from build123d import *

# Parameters (mm, degrees)
SKETCH2_R             = 19
BOSS_EXTRUDE1_DEPTH   = 5
SKETCH3_R             = 5
CUT_EXTRUDE1_DEPTH    = 43.679034666
SKETCH4_R             = 4
CUT_EXTRUDE2_DEPTH    = 43.679034666
M4X0_7_TAPPED_HOLE1_D = 3.3
CUT_EXTRUDE3_DEPTH    = 6.43
CIRPATTERN1_COUNT     = 4


with BuildPart() as part:
    # Sketch1 → Revolve1 (revolve)
    with BuildSketch(Plane(origin=(0, 0, 0), x_dir=(0, 0, -1), z_dir=(1, 0, 0)), mode=Mode.PRIVATE) as revolve1_sk:
        Polygon((0, 9), (0, 6.15), (26.545687362, 6.15), (28.453012328, 0), (29.5, 0), (27.011788484, 8.023017104), (25.5, 9), align=None)
    revolve(revolve1_sk.sketch.rotate(Axis((0, 9, 0), (0, -1, 0)), 180), axis=Axis((0, 9, 0), (0, -1, 0)))

    # Sketch2 → Boss-Extrude1 (add)
    with BuildSketch(Plane.XZ.offset(-6.15)):
        with Locations(Location((0, 0, 0), (0, 0, 90))):
            Circle(SKETCH2_R)
    extrude(amount=BOSS_EXTRUDE1_DEPTH)

    # Sketch3 → Cut-Extrude1 (cut, through all)
    with BuildSketch(Plane(origin=(0, 9, 0), x_dir=(1, 0, 0), z_dir=(0, 1, 0))):
        with Locations(Location((0, 19, 0), (0, 0, 270))):
            Circle(SKETCH3_R)
        with Locations(Location((19, 0, 0), (0, 0, 270))):
            Circle(SKETCH3_R)
        with Locations(Location((0, -19, 0), (0, 0, 270))):
            Circle(SKETCH3_R)
        with Locations(Location((-19, 0, 0), (0, 0, 270))):
            Circle(SKETCH3_R)
    extrude(amount=-CUT_EXTRUDE1_DEPTH, mode=Mode.SUBTRACT)

    # Sketch4 → Cut-Extrude2 (cut, through all)
    with BuildSketch(Plane(origin=(0, 9, 0), x_dir=(1, 0, 0), z_dir=(0, 1, 0))):
        with Locations(Location((0, 0, 0), (0, 0, 270))):
            Circle(SKETCH4_R)
    extrude(amount=-CUT_EXTRUDE2_DEPTH, mode=Mode.SUBTRACT)

    # M4x0.7 Tapped Hole1 (through all)
    with Locations(Plane(origin=(0, 9, 0), x_dir=(1, 0, 0), z_dir=(0, 1, 0))):
        with Locations((-15.556349186, 15.556349186), (15.556349186, 15.556349186), (15.556349186, -15.556349186), (-15.556349186, -15.556349186)):
            Hole(M4X0_7_TAPPED_HOLE1_D / 2)

    # Sketch9 → Cut-Extrude3 (cut)
    with BuildSketch(Plane.XY.offset(-29.5)):
        with BuildLine():
            Line((-9.875, 6.636508552), (9.875, 6.636508552))
            ThreePointArc((9.875, 6.636508552), (12.5, 4.011508552), (9.875, 1.386508552))
            Line((9.875, 1.386508552), (-9.875, 1.386508552))
            ThreePointArc((-9.875, 1.386508552), (-12.5, 4.011508552), (-9.875, 6.636508552))
        make_face()
    cut_extrude3 = extrude(amount=CUT_EXTRUDE3_DEPTH, mode=Mode.SUBTRACT)

    # CirPattern1: Cut-Extrude3 ×4 about axis
    cirpattern1_axis = Axis((0, 0, 0), (0, 1, 0))
    for i in range(1, CIRPATTERN1_COUNT):
        add(cut_extrude3.rotate(cirpattern1_axis, i * 360 / CIRPATTERN1_COUNT), mode=Mode.SUBTRACT)


solid = part.part
Build history of the part. All positions in model axes, mm. A direction names the side the tool comes from. Give positions to 0.01 mm unless a question says otherwise; leave off trailing zeros. Order: outer loops, then holes, each group sorted by start corner. A loop starts at its lowest first (then second) coordinate and runs counter-clockwise, first axis right, second up. Notation, with made-up numbers: M 10,2.5 L 25,2.5 A32 cw 25,39.5 Z; hole C 7,-8.75 d6. An arc over 180 degrees is marked long. Use one line per item in the form item = value.
Q1. Wall check: probe 1 along Z at (x, y) = (-15, 6.5); probe 2 along X at (y, z) = (5.75, 0); probe 3 along Y at (x, z) = (-21, 5). Give the ranges that are in metal, low to high.
Conclusion:
probe_1 = -23.03 to -17.11, -14 to -3, 3 to 14, 17.11 to 23.03
probe_2 = -14 to -4, 4 to 14
probe_3 = 6.15 to 9
Q2. Slice it at A-A, the plane y = 4.5. Write the cut outline in (x, z), and give its area (3 significant figures).
Conclusion:
outline = M -25.19,-12.45 A28.1 ccw -12.45,-25.19 L -12.45,-24.02 A27.06 cw -24.02,-12.45 Z; M -25.19,12.45 L -24.02,12.45 A27.06 cw -12.45,24.02 L -12.45,25.19 A28.1 ccw Z; M -18.34,-4.96 A19 ccw -4.96,-18.34 A5 cw 4.96,-18.34 A19 ccw 18.34,-4.96 A5 cw 18.34,4.96 A19 ccw 4.96,18.34 A5 cw -4.96,18.34 A19 ccw -18.34,4.96 A5 cw Z; M 12.45,-25.19 A28.1 ccw 25.19,-12.45 L 24.02,-12.45 A27.06 cw 12.45,-24.02 Z; M 12.45,24.02 A27.06 cw 24.02,12.45 L 25.19,12.45 A28.1 ccw 12.45,25.19 Z; hole C 0,0 d8
area = 1,010 mm2
Q3. Slice it at C-C, the plane x = 1. State how many separate pieces and enclosed holes the cut face has, and give its area (3 significant figures).
Conclusion:
separate_pieces = 6
enclosed_holes = 0
area = 177 mm2
Q4. Pull direction Z, two halves, no side cores. Call faces 1 (the cylindrical face through (24.741, 4.636, 12.425)), 2 (the conical face through (-1.193, 7.633, -27.106)), 3 (the flat face through (-0.1, 1.387, 28.3)): released by +Z, released by -Z, zero draft, split by the parting line, or undercut.
Conclusion:
face_1 = undercut
face_2 = split by the parting line
face_3 = zero draft
Q5. Pin check, flat tips, straight feed: P1, Ø10, axis at x = 6.5, z = 21, coming from the -Y side; P2, Ø2.5, axis at x = 1.5, z = 27.5, coming from the +Y side; P3, Ø1, axis at x = -5.5, y = 4, coming from the +Z side. Stop position of each tip, or through.
Conclusion:
P1 = 1.15
P2 = 8.49
P3 = 18.33
Q6. Which spindle directions (+Z, -Z, +X, -X, +Y, -Y) get a long thin tool onto all of the face, cutting with end or side? Do faces 4 (the flat face through (-25, 6.637, 0)), 5 (the flat face through (0.1, 1.387, -28.3)), 6 (the cylindrical face through (-13.53, 3.69, -13.34)), 7 (the cylindrical face through (12.434, 4.598, 24.899)). Say none if no direction does.
Conclusion:
face_4 = -X, -Y
face_5 = -Z, +Y
face_6 = -Y
face_7 = +Z
Q7. Slice it at B-B, the plane z = 0. Write the cut outline in (x, y), and give its area (3 significant figures).
Conclusion:
outline = M -29.5,0 L -28.45,0 L -28.02,1.39 L -29.07,1.39 Z; M -27.44,6.64 L -24,6.64 L -24,9 L -25.5,9 L -27.01,8.02 Z; M -14,1.15 L -4,1.15 L -4,9 L -14,9 Z; M 4,1.15 L 14,1.15 L 14,9 L 4,9 Z; M 24,6.64 L 27.44,6.64 L 27.01,8.02 L 25.5,9 L 24,9 Z; M 28.02,1.39 L 28.45,0 L 29.5,0 L 29.07,1.39 Z
area = 173 mm2
